from build123d import *

# Parameters (mm, degrees)
SKETCH1_W           = 390
SKETCH1_H           = 360
SKETCH1_R           = 2.1
SKETCH1_R_2         = 16
SKETCH1_R_3         = 2
SKETCH1_R_4         = 1.55
BOSS_EXTRUDE1_DEPTH = 6
CUT_EXTRUDE1_REACH  = 267.445
SKETCH5_W           = 390
SKETCH5_H           = 1
CUT_EXTRUDE2_DEPTH  = 266.444909539
CUT_EXTRUDE3_DEPTH  = 266.444909539


with BuildPart() as part:
    # Sketch1 → Boss-Extrude1 (new body)
    with BuildSketch(Plane(origin=(0, 0, 0), x_dir=(1, 0, 0), z_dir=(0, 1, 0))):
        Rectangle(SKETCH1_W, SKETCH1_H)
        with Locations(Location((-176, 161, 0), (0, 0, 270))):
            Circle(SKETCH1_R, mode=Mode.SUBTRACT)
        with Locations(Location((-176, -167, 0), (0, 0, 270))):
            Circle(SKETCH1_R, mode=Mode.SUBTRACT)
        with Locations(Location((-120, -90, 0), (0, 0, 270))):
            Circle(SKETCH1_R_2, mode=Mode.SUBTRACT)
        with Locations(Location((176, -167, 0), (0, 0, 90))):
            Circle(SKETCH1_R, mode=Mode.SUBTRACT)
        with Locations(Location((176, 161, 0), (0, 0, 90))):
            Circle(SKETCH1_R, mode=Mode.SUBTRACT)
        with Locations(Location((-160, -50, 0), (0, 0, 270))):
            Circle(SKETCH1_R_3, mode=Mode.SUBTRACT)
        with Locations(Location((-160, 100, 0), (0, 0, 270))):
            Circle(SKETCH1_R_3, mode=Mode.SUBTRACT)
        with Locations(Location((105, -50, 0), (0, 0, 270))):
            Circle(SKETCH1_R_3, mode=Mode.SUBTRACT)
        with Locations(Location((105, 100, 0), (0, 0, 270))):
            Circle(SKETCH1_R_3, mode=Mode.SUBTRACT)
        with Locations(Location((-119.684190721, -109.997506457, 0), (0, 0, 270))):
            Circle(SKETCH1_R_4, mode=Mode.SUBTRACT)
        with Locations(Location((-120.315809279, -70.002493543, 0), (0, 0, 270))):
            Circle(SKETCH1_R_4, mode=Mode.SUBTRACT)
        with Locations(Location((-173.106414611, -71.615200698, 0), (0, 0, 270))):
            Circle(SKETCH1_R_4, mode=Mode.SUBTRACT)
    extrude(amount=BOSS_EXTRUDE1_DEPTH)

    # Sketch4 → Cut-Extrude1 (cut, up to next)
    with BuildSketch(Plane(origin=(0, 6, 0), x_dir=(1, 0, 0), z_dir=(0, 1, 0)), mode=Mode.PRIVATE) as cut_extrude1_sk1:
        with BuildLine():
            Line((-135.998409614, -89.77441229), (-169.072254333, -78.302916757))
            Line((-169.072254333, -78.302916757), (-165.800861457, -68.853156465))
            Line((-165.800861457, -68.853156465), (-132.726704425, -80.303041999))
            ThreePointArc((-132.726704425, -80.303041999), (-104.876846958, -95.224006323), (-135.998409614, -89.77441229))
        make_face()
    cut_extrude1_tool1 = extrude(cut_extrude1_sk1.sketch, amount=-CUT_EXTRUDE1_REACH, mode=Mode.PRIVATE) & part.part
    add(cut_extrude1_tool1.solids().sort_by_distance((-129.350351, 6, 86.764679))[0], mode=Mode.SUBTRACT)

    # Sketch5 → Cut-Extrude2 (cut, through all)
    with BuildSketch(Plane(origin=(0, 6, 0), x_dir=(1, 0, 0), z_dir=(0, 1, 0))):
        with Locations((0, -179.5)):
            Rectangle(SKETCH5_W, SKETCH5_H)
    extrude(amount=-CUT_EXTRUDE2_DEPTH, mode=Mode.SUBTRACT)

    # Sketch6 → Cut-Extrude3 (cut, through all)
    with BuildSketch(Plane(origin=(0, 6, 0), x_dir=(1, 0, 0), z_dir=(0, 1, 0))):
        Polygon((195, -179), (195, 180), (-195, 180), (-195, -179), (-194, -179), (-194, 179), (194, 179), (194, -179), align=None)
    extrude(amount=-CUT_EXTRUDE3_DEPTH, mode=Mode.SUBTRACT)


solid = part.part
The listing builds one solid part. Answer for the finished solid, in the listing's coordinates (mm). A direction names the side the tool comes from. Give positions to 0.01 mm unless a question says otherwise; leave off trailing zeros. Answer as a JSON object with one key per item and string values.
1. Find the intervals of material crossed by L1, parallel to Z at x = 176, y = 3.8; L2, parallel to X at y = 1.9, z = 167; L3, parallel to Z at x = -120, y = 4.15 (3 decimals), in increasing order. Write a range as [from, to].
Determined:
{"L1": "[-179, -163.1], [-158.9, 164.9], [169.1, 179]", "L2": "[-194, -178.1], [-173.9, 173.9], [178.1, 194]", "L3": "[-179, 68.485], [71.52, 74], [106, 108.48], [111.515, 179]"}
2. For faces 3 (the flat face through (-149.495, 3.042, 74.498)), 4 (the flat face through (-3, 6, -3)), determine the directions among +Z, -Z, +X, -X, +Y, -Y from which every point of the face is accessible in a straight line to the end or side of a thin tool.
Determined:
{"face 3": "+Y, -Y", "face 4": "+Z, -Z, +X, -X, +Y"}
3. A flat-ended cylindrical pin translates along its axis: pin 1 Ø2.5 at (x, z) = (-173.11, 71.62) entering from -Y. Find the tip coordinate at first contact, or state that the pin passes through.
Determined:
{"pin 1": "through"}
4. For a pull along X with two mould halves and no side action, classify faces 1 (the flat face through (-152.3, 3.04, 84.12)), 2 (the flat face through (-3, 0, -3)) as pulls with the +X half, pulls with the -X half, needs draft (parallel to the pull), parting line crosses it, or undercut.
Determined:
{"face 1": "undercut", "face 2": "needs draft"}
